Design review of the part built by this model. Coordinates are the model's own, in mm. Face numbers are marked on the shaded views. Give positions to 0.01 mm unless a question says otherwise; leave off trailing zeros. Write each loop counter-clockwise with the first axis right and the second up, starting at its lowest first coordinate (ties: lowest second). Pieces come first, ordered by that corner, then holes.
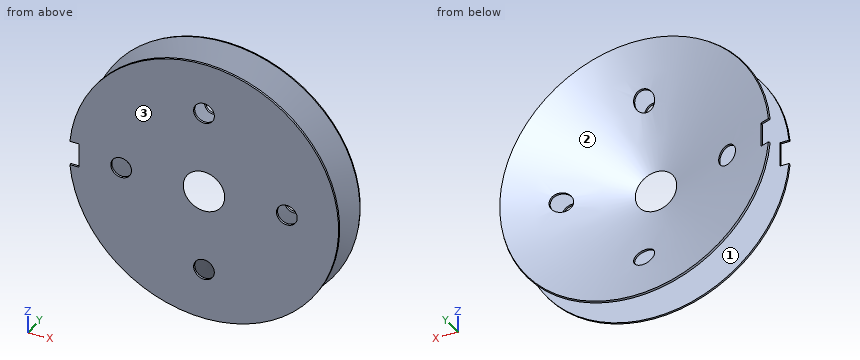
```python
from build123d import *

# Parameters (mm, degrees)
SKETCH2_R          = 5
SKETCH2_W          = 10
SKETCH2_H          = 11.93656
CUT_EXTRUDE1_DEPTH = 95.551012926


with BuildPart() as part:
    # Sketch1 → Revolve-Thin1 (revolve)
    with BuildSketch(Plane.XY):
        Polygon((-65, 0), (-10, -20.018362885), (-65, -20.018362885), (-65, -19.018362885), (-15.67128182, -19.018362885), (-65.342020143, -0.939692621), align=None)
    revolve(axis=Axis((0, 0, 0), (0, -1, 0)))

    # Sketch2 → Cut-Extrude1 (cut, through all)
    with BuildSketch(Plane(origin=(0, 0, 0), x_dir=(1, 0, 0), z_dir=(0, 1, 0))):
        with Locations(Location((-40, 0, 0), (0, 0, 270))):
            Circle(SKETCH2_R)
        with Locations(Location((0, 40, 0), (0, 0, 270))):
            Circle(SKETCH2_R)
        with Locations(Location((40, 0, 0), (0, 0, 270))):
            Circle(SKETCH2_R)
        with Locations(Location((0, -40, 0), (0, 0, 270))):
            Circle(SKETCH2_R)
        with Locations((-65.342020143, 0)):
            Rectangle(SKETCH2_W, SKETCH2_H)
    extrude(amount=-CUT_EXTRUDE1_DEPTH, mode=Mode.SUBTRACT)


solid = part.part
```
(1) To check wall thickness, follow L1, parallel to Y at x = 30.5, z = -7.5; L2, parallel to Y at x = -41, z = 17; L3, parallel to X at y = -19.7, z = -40. State the ranges of each line that lie inside material, in increasing order.
Resolved:
L1: y = -20.02 to -19.02, -13.29 to -12.23
L2: y = -20.02 to -19.02, -8.57 to -7.5
L3: x = -51.23 to -5, 5 to 51.23
(2) Mouldability with a two-part tool opening along Y and no side actions: class the marked faces 1, 2 and 3 as pulls with the +Y half, pulls with the -Y half, needs draft (parallel to the pull), parting line crosses it, or undercut.
Resolved:
face 1: undercut
face 2: pulls with the +Y half
face 3: pulls with the -Y half
(3) Clearance check with flat-ended pins moving along their axes: P1, Ø1.1, axis at y = -19.5, z = -2.5, coming from the -X side; P2, Ø6, axis at x = 40, z = 0, coming from the +Y side; P3, Ø5, axis at x = -52, z = -24, coming from the +Y side; P4, Ø8, axis at y = -17.5, z = 41.5, coming from the +X side. State where each tip first meets the part, or that it passes through.
Resolved:
P1: stops at x = -60.34
P2: passes through
P3: stops at y = -1.9
P4: stops at x = 52.88
(4) Consider section B-B, the plane x = -40. Give the number of separate pieces and of enclosed holes in the cut face, then the cut area to 3 significant figures.
Resolved:
separate pieces: 4
enclosed holes: 0
area: 191 mm2
(5) Consider section D-D, the plane y = -4.75. Give the boundary of the cut face in (x, z).
Resolved:
outline: circle Ø109.75 at (0, 0); hole circle Ø103.9 at (0, 0)
(6) Consider section A-A, the plane z = 0. Give the boundary of the cut face in (x, y), then the cut area to 3 significant figures.
Resolved:
outline: (-60.34, -20.02) - (-45, -20.02) - (-45, -19.02) - (-60.34, -19.02) - close; (-60.34, -2.76) - (-45, -8.34) - (-45, -7.28) - (-60.34, -1.7) - close; (-35, -20.02) - (-10, -20.02) - (-35, -10.92) - (-35, -11.98) - (-15.67, -19.02) - (-35, -19.02) - close; (10, -20.02) - (35, -20.02) - (35, -19.02) - (15.67, -19.02) - (35, -11.98) - (35, -10.92) - close; (45, -20.02) - (65, -20.02) - (65, -19.02) - (45, -19.02) - close; (45, -8.34) - (65.34, -0.94) - (65, 0) - (45, -7.28) - close
area: 165 mm2
